from build123d import *

# Parameters (mm, degrees)
F1_DEPTH = 5.08
F2_DEPTH = 5.08
F3_W     = 124.8834840953
F3_H     = 134.0803280473
F4_DEPTH = 25.4
F5_DEPTH = 1.27
F6_DEPTH = 1.27


with BuildPart() as f1:
    # F0 (on Front) → F1 (new body)
    with BuildSketch(Plane.XZ):
        with BuildLine():
            add(Edge.make_bspline(
                [(11.6870266183, 8.3659507286), (11.9476031572, 8.1243832132), (12.5616108346, 7.4348870399), (13.3502602627, 5.9055860485), (12.8304196463, 2.6136928469), (12.1032885822, -3.9726756525), (11.7671016032, -8.6546761386), (11.3077259518, -11.7183290107), (11.0820746049, -13.2232354954)],
                knots=[0.7644347581, 0.7644347581, 0.7644347581, 0.7644347581, 0.7813803339, 0.8102561854, 0.8494051355, 0.9057589485, 0.9537075591, 1, 1, 1, 1], degree=3))
            Line((11.6870266183, 8.3659507286), (10.7098612934, -7.1798651479))
            Line((10.7098612934, -7.1798651479), (-10.6029463932, 18.994666636))
            Line((-10.6029463932, 18.994666636), (-7.8187826003, 81.9431145827))
            add(Edge.make_bspline(
                [(-10.6029463932, 84.9773436785), (-9.8645957866, 84.411917966), (-8.8470388386, 83.6326772405), (-8.0272766718, 82.3316307612), (-7.8187826003, 81.9431145827)],
                knots=[0, 0, 0, 0, 0.0369842854, 0.0509698458, 0.0509698458, 0.0509698458, 0.0509698458], degree=3))
            add(Edge.make_bspline(
                [(-11.1952358857, -13.2855195552), (-11.1963398761, -12.8902117283), (-11.1997561984, -11.6669231231), (-11.1512885463, -5.3731858959), (-11.3422819981, 1.4393792063), (-12.1461643066, 4.6189611976), (-13.2850553088, 9.1238655935), (-15.2318124981, 13.6348809881), (-16.5294824008, 17.2010053959), (-19.3261405399, 23.6368379744), (-19.7379489625, 26.452730971), (-18.8574929103, 31.5305578619), (-16.6797816611, 35.2468825016), (-14.5909185063, 40.6408371255), (-13.4119591393, 46.1621954132), (-12.5394588361, 53.3896491248), (-12.0546254183, 59.9791874234), (-12.4642284532, 65.9827168693), (-12.3457592591, 73.9226808987), (-11.3164428193, 80.5227149139), (-11.5649092387, 84.7450814286), (-10.8268692537, 84.9232783602), (-10.6029463932, 84.9773436785)],
                knots=[0, 0, 0, 0, 0.0273896804, 0.0847579572, 0.1451631407, 0.1862204743, 0.2349457062, 0.2850522094, 0.3309978555, 0.390291, 0.4296935499, 0.4796750401, 0.527816225, 0.5818528524, 0.6365092781, 0.6980539867, 0.7565756752, 0.8124783975, 0.8767822708, 0.9378286387, 0.9811370802, 1, 1, 1, 1], degree=3))
            Line((-11.1952358857, -13.2855195552), (10.8409429303, -13.2855195552))
            add(Edge.make_bspline(
                [(10.8409429303, -13.2855195552), (10.9216527758, -13.2575733481), (11.0020770139, -13.2366740148), (11.0820746049, -13.2232354954)],
                knots=[0.9988692567, 0.9988692567, 0.9988692567, 0.9988692567, 1, 1, 1, 1], degree=3))
        make_face()
        with BuildLine():
            Line((10.7098612934, -7.1798651479), (11.6870266183, 8.3659507286))
            add(Edge.make_bspline(
                [(-7.8187826003, 81.9431145827), (-7.3326835412, 81.037298185), (-6.246332701, 78.0877738667), (-5.7619281696, 71.7972152113), (-5.7903461619, 61.0472196354), (-5.6098025476, 47.5528084715), (-5.6232359348, 35.7951775922), (-6.6035814728, 31.5572406566), (-6.642373723, 26.8588973108), (-4.7217209893, 21.7576733197), (-2.3324429206, 17.8568763905), (-0.0644904347, 14.9988475653), (2.1698029367, 12.9502128359), (5.7523840475, 11.2499433455), (8.6363164493, 10.2542124123), (10.6765655712, 9.2073747067), (11.4911211984, 8.5475648745), (11.6870266183, 8.3659507286)],
                knots=[0.0509698458, 0.0509698458, 0.0509698458, 0.0509698458, 0.0835768534, 0.1402547932, 0.2115954168, 0.293701069, 0.3674969806, 0.4121442254, 0.4580916534, 0.50894046, 0.5557476766, 0.5967458601, 0.6345135251, 0.6775157549, 0.7161326985, 0.7516948155, 0.7644347581, 0.7644347581, 0.7644347581, 0.7644347581], degree=3))
            Line((-7.8187826003, 81.9431145827), (-10.6029463932, 18.994666636))
            Line((-10.6029463932, 18.994666636), (10.7098612934, -7.1798651479))
        make_face()
        with BuildLine():
            Line((11.0820746049, -15.9663576633), (11.0820746049, -13.2855195552))
            Line((11.0820746049, -13.2855195552), (10.8409429303, -13.2855195552))
            add(Edge.make_bspline(
                [(8.3953980002, -15.9663576633), (9.1364610409, -14.6227373643), (10.004055933, -13.5752960653), (10.8409429303, -13.2855195552)],
                knots=[0.9871444865, 0.9871444865, 0.9871444865, 0.9871444865, 0.9988692567, 0.9988692567, 0.9988692567, 0.9988692567], degree=3))
            Line((8.3953980003, -15.9663576633), (11.0820746049, -15.9663576633))
        make_face()
        with BuildLine():
            add(Edge.make_bspline(
                [(8.3953980002, -15.9663576633), (9.1364610409, -14.6227373643), (10.004055933, -13.5752960653), (10.8409429303, -13.2855195552)],
                knots=[0.9871444865, 0.9871444865, 0.9871444865, 0.9871444865, 0.9988692567, 0.9988692567, 0.9988692567, 0.9988692567], degree=3))
            Line((10.8409429303, -13.2855195552), (-11.1952358857, -13.2855195552))
            Line((-11.1952358857, -13.2855195552), (-11.0308257863, -15.9663576633))
            Line((-11.0308257863, -15.9663576633), (8.3953980003, -15.9663576633))
        make_face()
        with BuildLine():
            Line((11.0820746049, -13.2855195552), (11.0820746049, -13.2232354954))
            add(Edge.make_bspline(
                [(10.8409429303, -13.2855195552), (10.9216527758, -13.2575733481), (11.0020770139, -13.2366740148), (11.0820746049, -13.2232354954)],
                knots=[0.9988692567, 0.9988692567, 0.9988692567, 0.9988692567, 1, 1, 1, 1], degree=3))
            Line((10.8409429303, -13.2855195552), (11.0820746049, -13.2855195552))
        make_face()
    extrude(amount=F1_DEPTH)

    # F2 (add): a face of the model
    f2_faces = [f1.faces().sort_by_distance(p)[0] for p in [
        (-5.0809274024, 0, 19.1888153538),
    ]]
    extrude(f2_faces, amount=F2_DEPTH)

    # F3 (on face) → F4 (cut)
    with BuildSketch(Plane.XZ.offset(5.08)):
        with Locations((7.2313416749, 30.1963053644)):
            Rectangle(F3_W, F3_H)
        with BuildLine():
            Line((-11.0308257863, -15.9663576633), (-11.1952358857, -13.2855195552))
            add(Edge.make_bspline(
                [(-11.1952358857, -13.2855195552), (-11.1963398761, -12.8902117283), (-11.1997561984, -11.6669231231), (-11.1512885463, -5.3731858959), (-11.3422819981, 1.4393792063), (-12.1461643066, 4.6189611976), (-13.2850553088, 9.1238655935), (-15.2318124981, 13.6348809881), (-16.5294824008, 17.2010053959), (-19.3261405399, 23.6368379744), (-19.7379489625, 26.452730971), (-18.8574929103, 31.5305578619), (-16.6797816611, 35.2468825016), (-14.5909185063, 40.6408371255), (-13.4119591393, 46.1621954132), (-12.5394588361, 53.3896491248), (-12.0546254183, 59.9791874234), (-12.4642284532, 65.9827168693), (-12.3457592591, 73.9226808987), (-11.3164428193, 80.5227149139), (-11.5649092387, 84.7450814286), (-10.8268692537, 84.9232783602), (-10.6029463932, 84.9773436785)],
                knots=[0, 0, 0, 0, 0.0273896804, 0.0847579572, 0.1451631407, 0.1862204743, 0.2349457062, 0.2850522094, 0.3309978555, 0.390291, 0.4296935499, 0.4796750401, 0.527816225, 0.5818528524, 0.6365092781, 0.6980539867, 0.7565756752, 0.8124783975, 0.8767822708, 0.9378286387, 0.9811370802, 1, 1, 1, 1], degree=3))
            add(Edge.make_bspline(
                [(11.0820746049, -13.2232354954), (11.3077259518, -11.7183290107), (11.7671016032, -8.6546761386), (12.1032885822, -3.9726756525), (12.8304196463, 2.6136928469), (13.3502602627, 5.9055860485), (12.443365527, 7.6641811468), (11.0743289472, 9.0032850711), (8.6363164493, 10.2542124123), (5.7523840475, 11.2499433455), (2.1698029367, 12.9502128359), (-0.0644904347, 14.9988475653), (-2.3324429206, 17.8568763905), (-4.7217209893, 21.7576733197), (-6.642373723, 26.8588973108), (-6.6035814728, 31.5572406566), (-5.6232359348, 35.7951775922), (-5.6098025476, 47.5528084715), (-5.7903461619, 61.0472196354), (-5.7619281696, 71.7972152113), (-6.2885094778, 78.6354885776), (-8.1960757736, 83.1341725308), (-9.8645957866, 84.411917966), (-10.6029463932, 84.9773436785)],
                knots=[0.7644347581, 0.7644347581, 0.7644347581, 0.7644347581, 0.810727199, 0.8586758096, 0.9150296226, 0.9541785727, 0.9830544242, 1.0127399426, 1.0483020596, 1.0869190032, 1.1299212329, 1.167688898, 1.2086870814, 1.2554942981, 1.3063431047, 1.3522905327, 1.3969377775, 1.470733689, 1.5528393413, 1.6241799649, 1.6808579047, 1.7274504726, 1.7644347581, 1.7644347581, 1.7644347581, 1.7644347581], degree=3))
            Line((11.0820746049, -13.2232354954), (11.0820746049, -15.9663576633))
            Line((11.0820746049, -15.9663576633), (-11.0308257863, -15.9663576633))
        make_face(mode=Mode.SUBTRACT)
        with BuildLine():
            add(Edge.make_bspline(
                [(-11.1952358857, -13.2855195552), (-11.1963398761, -12.8902117283), (-11.1997561984, -11.6669231231), (-11.1512885463, -5.3731858959), (-11.3422819981, 1.4393792063), (-12.1461643066, 4.6189611976), (-13.2850553088, 9.1238655935), (-15.2318124981, 13.6348809881), (-16.5294824008, 17.2010053959), (-19.3261405399, 23.6368379744), (-19.7379489625, 26.452730971), (-18.8574929103, 31.5305578619), (-16.6797816611, 35.2468825016), (-14.5909185063, 40.6408371255), (-13.4119591393, 46.1621954132), (-12.5394588361, 53.3896491248), (-12.0546254183, 59.9791874234), (-12.4642284532, 65.9827168693), (-12.3457592591, 73.9226808987), (-11.3164428193, 80.5227149139), (-11.5649092387, 84.7450814286), (-10.8268692537, 84.9232783602), (-10.6029463932, 84.9773436785)],
                knots=[0, 0, 0, 0, 0.0273896804, 0.0847579572, 0.1451631407, 0.1862204743, 0.2349457062, 0.2850522094, 0.3309978555, 0.390291, 0.4296935499, 0.4796750401, 0.527816225, 0.5818528524, 0.6365092781, 0.6980539867, 0.7565756752, 0.8124783975, 0.8767822708, 0.9378286387, 0.9811370802, 1, 1, 1, 1], degree=3))
            Line((-11.1952358857, -13.2855195552), (-11.0308257863, -15.9663576633))
            Line((-11.0308257863, -15.9663576633), (11.0820746049, -15.9663576633))
            Line((11.0820746049, -15.9663576633), (11.0820746049, -13.2232354954))
            add(Edge.make_bspline(
                [(11.0820746049, -13.2232354954), (11.3077259518, -11.7183290107), (11.7671016032, -8.6546761386), (12.1032885822, -3.9726756525), (12.8304196463, 2.6136928469), (13.3502602627, 5.9055860485), (12.443365527, 7.6641811468), (11.0743289472, 9.0032850711), (8.6363164493, 10.2542124123), (5.7523840475, 11.2499433455), (2.1698029367, 12.9502128359), (-0.0644904347, 14.9988475653), (-2.3324429206, 17.8568763905), (-4.7217209893, 21.7576733197), (-6.642373723, 26.8588973108), (-6.6035814728, 31.5572406566), (-5.6232359348, 35.7951775922), (-5.6098025476, 47.5528084715), (-5.7903461619, 61.0472196354), (-5.7619281696, 71.7972152113), (-6.2885094778, 78.6354885776), (-8.1960757736, 83.1341725308), (-9.8645957866, 84.411917966), (-10.6029463932, 84.9773436785)],
                knots=[0.7644347581, 0.7644347581, 0.7644347581, 0.7644347581, 0.810727199, 0.8586758096, 0.9150296226, 0.9541785727, 0.9830544242, 1.0127399426, 1.0483020596, 1.0869190032, 1.1299212329, 1.167688898, 1.2086870814, 1.2554942981, 1.3063431047, 1.3522905327, 1.3969377775, 1.470733689, 1.5528393413, 1.6241799649, 1.6808579047, 1.7274504726, 1.7644347581, 1.7644347581, 1.7644347581, 1.7644347581], degree=3))
        make_face()
        Polygon((-7.6687936671, 0), (0, 12.9914516583), (7.6687936671, 0), (0, -13.0022913218), align=None, mode=Mode.SUBTRACT)
    extrude(amount=-F4_DEPTH, mode=Mode.SUBTRACT)

    # F5 (add): a face of the model
    f5_faces = [f1.faces().sort_by_distance(p)[0] for p in [
        (0, -5.08, -0.0036132211),
    ]]
    extrude(f5_faces, amount=F5_DEPTH)

    # F6 (add): a face of the model
    f6_faces = [f1.faces().sort_by_distance(p)[0] for p in [
        (0, 5.08, -0.0036132211),
    ]]
    extrude(f6_faces, amount=F6_DEPTH)


solid = f1.part
Could you check a few things on this model? Use its own coordinates, in mm. Give positions to 0.01 mm unless a question says otherwise; leave off trailing zeros. Order: outer loops, then holes, each group sorted by start corner. A loop starts at its lowest first (then second) coordinate and runs counter-clockwise, first axis right, second up. Notation, with made-up numbers: (70.5, 81.25) -> (110.5, 81.25) arc R20 ccw to (110.5, 118.25) -> close; hole circle Ø4 at (40, 9). An arc over 180 degrees is marked (long way). Answer in a Markdown table with one row per item. Add a question column.
Item 1: Please list where these lines run through material, in increasing order: probe 1 along Z at (x, y) = (5.25, 5); probe 2 along X at (y, z) = (-1.5, 11.25); probe 3 along X at (y, z) = (5.75, -1).
Item 2: Imagine slicing it at B-B (x = 3.5). List the corners of the cut face in (y, z) for me.
Item 3: Imagine slicing it at A-A (y = -1). List the corners of the cut face in (x, z) for me, and give its area (3 significant figures).
Item 4: I'm going to push flat-ended pins straight in: P1, Ø3, axis at x = 5, y = 3.5, coming from the -Z side; P2, Ø1, axis at x = 4.5, y = 2, coming from the +Z side. Where does each tip first touch, or does it pass through?
Result:
| question | item | result |
|---|---|---|
| 1 | probe 1 | -4.1 to 4.1 |
| 1 | probe 2 | -1.03 to 1.03 |
| 1 | probe 3 | -7.08 to 7.08 |
| 2 | outline | (-6.35, -7.07) -> (6.35, -7.07) -> (6.35, 7.06) -> (-6.35, 7.06) -> close |
| 3 | outline | (-7.67, 0) -> (0, -13) -> (7.67, 0) -> (0, 12.99) -> close |
| 3 | area | 199 mm2 |
| 4 | P1 | z = -7.07 |
| 4 | P2 | z = 6.22 |
